Input: dimensioned drawing with shaded views. Units: mm. Origin: part minimum x, y, z. A direction names the side the tool comes from. Give positions to 0.01 mm unless a question says otherwise; leave off trailing zeros. Order: outer loops, then holes, each group sorted by start corner. A loop starts at its lowest first (then second) coordinate and runs counter-clockwise, first axis right, second up.
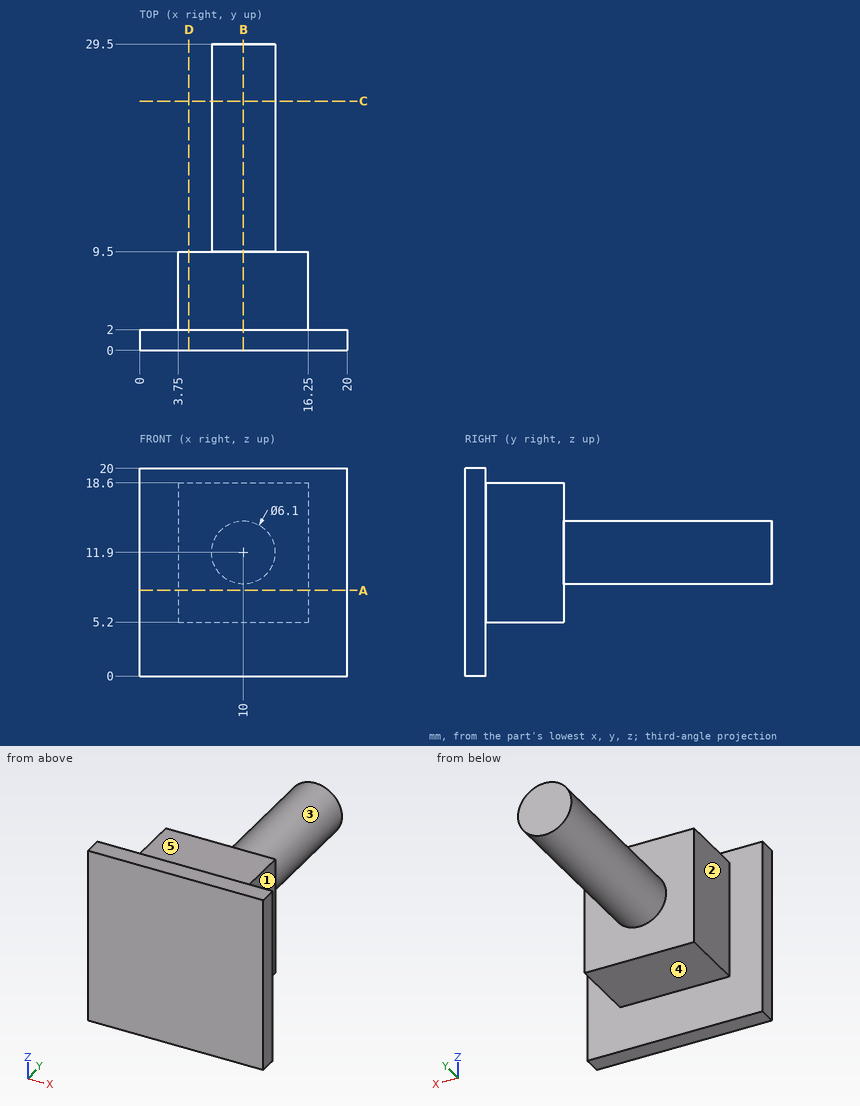
1) Section query D-D, the plane x = 4.75. Return the cut outline in (y, z).
Report:
outline: (0, 0) - (2, 0) - (2, 5.2) - (9.5, 5.2) - (9.5, 18.6) - (2, 18.6) - (2, 20) - (0, 20) - close
2) Section query B-B, the plane x = 10. Return the cut outline in (y, z).
Report:
outline: (0, 0) - (2, 0) - (2, 5.2) - (9.5, 5.2) - (9.5, 8.85) - (29.5, 8.85) - (29.5, 14.95) - (9.5, 14.95) - (9.5, 18.6) - (2, 18.6) - (2, 20) - (0, 20) - close
3) Reachability of the marked faces 1, 2, 3, 4 and 5 from +Z, -Z, +X, -X, +Y, -Y: full face, straight path, thin tool, end or side. Return the list, or none.
Report:
face 1: +Z, -Z, +X, +Y
face 2: +Z, -Z, -X, +Y
face 3: +Y
face 4: -Z, +X, -X, +Y
face 5: +Z, +X, -X, +Y
4) Section query A-A, the plane z = 8.25. Return the cut outline in (x, y).
Report:
outline: (0, 0) - (20, 0) - (20, 2) - (16.25, 2) - (16.25, 9.5) - (3.75, 9.5) - (3.75, 2) - (0, 2) - close
5) Material intervals for L1, parallel to Z at x = 12, y = 6.5; L2, parallel to Y at x = 17.5, z = 12.25; L3, parallel to X at y = 6.75, z = 14.25, sorted ascending.
Report:
L1: z = 5.2 to 18.6
L2: y = 0 to 2
L3: x = 3.75 to 16.25
6) Pin query (flat end, axial travel): pin 1 (3 mm diameter, centred on y = 22.5, z = 8, fed in from -X); pin 2 (12 mm diameter, centred on x = 5.5, y = 10, fed in from -Z); pin 3 (4 mm diameter, centred on x = 8, y = 7, fed in from +Z). Return the tip coordinate at first contact, or that it passes through.
Report:
pin 1: stops at x = 8.12
pin 2: stops at z = 5.2
pin 3: stops at z = 18.6
7) Section query C-C, the plane y = 24. Return the cut outline in (x, z).
Report:
outline: circle Ø6.1 at (10, 11.9)
